```python
from build123d import *

# Parameters (mm, degrees)
BOSS_EXTRUDE1_DEPTH = 5
SKETCH3_R           = 1.5
CUT_EXTRUDE3_DEPTH  = 126.099960032
FILLET1_R           = 5
FILLET2_R           = 5
FILLET3_R           = 5
FILLET4_R           = 5
FILLET5_R           = 5
FILLET6_R           = 5


with BuildPart() as part:
    # Sketch1 → Boss-Extrude1 (new body)
    with BuildSketch(Plane.XY):
        Polygon((0, 40), (30, 10), (70, 10), (100, 40), (100, 75), (0, 75), align=None)
    extrude(amount=BOSS_EXTRUDE1_DEPTH)

    # Sketch3 → Cut-Extrude3 (cut, through all)
    with BuildSketch(Plane.XY.offset(5)):
        with Locations((50, 20)):
            Circle(SKETCH3_R)
        with Locations((85, 63)):
            Circle(SKETCH3_R)
        with Locations((15, 63)):
            Circle(SKETCH3_R)
        with BuildLine():
            Line((35, 49.5), (65, 49.5))
            ThreePointArc((65, 49.5), (73, 41.5), (65, 33.5))
            Line((65, 33.5), (35, 33.5))
            ThreePointArc((35, 33.5), (27, 41.5), (35, 49.5))
        make_face()
    extrude(amount=-CUT_EXTRUDE3_DEPTH, mode=Mode.SUBTRACT)

    # Fillet1
    fillet1_edges = [part.edges().sort_by_distance(p)[0] for p in [
        (0, 40, 2.5),
    ]]
    fillet(fillet1_edges, radius=FILLET1_R)

    # Fillet2
    fillet2_edges = [part.edges().sort_by_distance(p)[0] for p in [
        (100, 40, 2.5),
    ]]
    fillet(fillet2_edges, radius=FILLET2_R)

    # Fillet3
    fillet3_edges = [part.edges().sort_by_distance(p)[0] for p in [
        (70, 10, 2.5),
    ]]
    fillet(fillet3_edges, radius=FILLET3_R)

    # Fillet4
    fillet4_edges = [part.edges().sort_by_distance(p)[0] for p in [
        (30, 10, 2.5),
    ]]
    fillet(fillet4_edges, radius=FILLET4_R)

    # Fillet5
    fillet5_edges = [part.edges().sort_by_distance(p)[0] for p in [
        (100, 75, 2.5),
    ]]
    fillet(fillet5_edges, radius=FILLET5_R)

    # Fillet6
    fillet6_edges = [part.edges().sort_by_distance(p)[0] for p in [
        (0, 75, 2.5),
    ]]
    fillet(fillet6_edges, radius=FILLET6_R)


solid = part.part
```
Could you check a few things on this model? Use its own coordinates, in mm. Round coordinates to 2 decimals unless told otherwise and drop trailing zeros. Loops run counter-clockwise (first coordinate to the right, second up) from the corner with the lowest first, then second, coordinate; pieces in that order, holes last. Notation, with made-up numbers: (87.5, 11.5) - (121.5, 11.5) arc R22 ccw to (121.5, 38.5) - close; hole circle Ø7 at (78, 40.5). An arc over 180 degrees is marked (long way). Answer in a Markdown table with one row per item. Add a question column.
(1) I'm going to push flat-ended pins straight in: pin 1 (1.8 mm diameter, centred on x = 50, y = 20, fed in from -Z); pin 2 (4 mm diameter, centred on x = 15, y = 63, fed in from +Z). Where does each tip first touch, or does it pass through?
(2) If we section it at C-C (z = 4.15): Please give me the cut outline in (x, y).
(3) If we mould it in two halves opening along X, with no side actions, what happens to faces 1 (the face through (100, 56, 2)), 2 (the face through (50, 33.5, 3)), 3 (the face through (2, 74, 3)), 4 (the face through (50, 49.5, 3))? For each: pulls with the +X half, pulls with the -X half, needs draft (parallel to the pull), parting line crosses it, or undercut.
(4) If we section it at A-A (y = 20): Please give me the cut outline in (x, z), plus the area to 3 significant figures.
(5) If we section it at B-B (x = 85): Please give me the cut outline in (y, z), plus the area to 3 significant figures.
(6) I need wall thicknesses on line 1 along Y through (x, z) = (61, 4.2); line 2 along Y through (x, z) = (49, 1.7); line 3 along Y through (x, z) = (85, 1.8). Which ranges of each line are inside material? Lowest first, please.
Model answer:
| question | item | result |
|---|---|---|
| 1 | pin 1 | passes through |
| 1 | pin 2 | stops at z = 5 |
| 2 | outline | (0, 42.07) arc R5 ccw to (1.46, 38.54) - (28.54, 11.46) arc R5 ccw to (32.07, 10) - (67.93, 10) arc R5 ccw to (71.46, 11.46) - (98.54, 38.54) arc R5 ccw to (100, 42.07) - (100, 70) arc R5 ccw to (95, 75) - (5, 75) arc R5 ccw to (0, 70) - close; hole circle Ø3 at (15, 63); hole (35, 33.5) - (65, 33.5) arc R8 ccw to (65, 49.5) - (35, 49.5) arc R8 ccw to start; hole circle Ø3 at (50, 20); hole circle Ø3 at (85, 63) |
| 3 | face 1 | pulls with the +X half |
| 3 | face 2 | undercut |
| 3 | face 3 | pulls with the -X half |
| 3 | face 4 | undercut |
| 4 | outline | (20, 0) - (48.5, 0) - (48.5, 5) - (20, 5) - close; (51.5, 0) - (80, 0) - (80, 5) - (51.5, 5) - close |
| 4 | area | 285 mm² |
| 5 | outline | (25, 0) - (61.5, 0) - (61.5, 5) - (25, 5) - close; (64.5, 0) - (75, 0) - (75, 5) - (64.5, 5) - close |
| 5 | area | 235 mm² |
| 6 | line 1 | y = 10 to 33.5, 49.5 to 75 |
| 6 | line 2 | y = 10 to 18.88, 21.12 to 33.5, 49.5 to 75 |
| 6 | line 3 | y = 25 to 61.5, 64.5 to 75 |
